Model file for the job. Use its own axes, mm. A direction names the side the tool comes from. Round coordinates to 2 decimals unless told otherwise and drop trailing zeros. Order: outer loops, then holes, each group sorted by start corner. A loop starts at its lowest first (then second) coordinate and runs counter-clockwise, first axis right, second up. Notation, with made-up numbers: (53, 68) - (106, 68) arc R17 ccw to (106, 84) - close; hole circle Ø6 at (-16.75, 88.25). An arc over 180 degrees is marked (long way). Answer as CSV lines item,"result". Start each with the question number.
1. Wall check: line 1 along Y through (x, z) = (31, 2.5); line 2 along Y through (x, z) = (-102.82, 1); line 3 along X through (y, z) = (21.5, 3.35). Give the ranges that are in metal, low to high. Write a range as [from, to].
2. Pull direction Y, two halves, no side cores. Call faces 1 (the face through (104.2, 13.6, 2)), 2 (the face through (33.03, 17, 2)), 3 (the face through (-9, 1, 0)): released by +Y, released by -Y, zero draft, split by the parting line, or undercut.
3. Band-saw the part on B-B on x = -37. List the corners of the cut face in (y, z), then the cut area to 3 significant figures.
4. Band-saw the part on A-A on x = -63.55. List the corners of the cut face in (y, z) (3 decimals), then the cut area to 3 significant figures.
5. Pin check, flat tip, straight feed: pin 1 Ø6 at (x, y) = (102.82, 15) entering from +Z. Stop position of the tip, or through.
6. Band-saw the part on C-C on z = 0.75. State how many separate pieces and enclosed holes the cut face has, then the cut area to 3 significant figures.
7. 3-axis set-ups, long thin cutter, end or side, ignore diameter. For faces 4 (the face through (-33.03, 18, 2)), 5 (the face through (-111, 23, 2)), 6 (the face through (-101, 28, 2)): which of +Z, -Z, +X, -X, +Y, -Y reach the whole face in a straight line?
8. Band-saw the part on D-D on x = 68. List the corners of the cut face in (y, z).
Autodesk Fusion 360 part; units mm, degrees
sketch "Sketch1" plane through (0, 0, 0) normal (0, 0, 1) x (1, 0, 0)
  line L0 (-111, 0.4) -> (111, 0.4)
  line L1 (111, 0.4) -> (111, 44.05)
  line L2 (111, 44.05) -> (-111, 44.05)
  line L3 (-111, 44.05) -> (-111, 0.4)
extrude "Extrude1" add sketch "Sketch1" along normal blind 4
sketch "Sketch2" plane through (0, 0, 0) normal (0, 0, 1) x (1, 0, 0)
  circle A0 centre (-63.55, 22.225) radius 19.5
  circle A1 centre (-79.55, 6.225) radius 1.8
  circle A2 centre (-79.55, 38.225) radius 1.8
  circle A3 centre (-47.55, 6.225) radius 1.8
  circle A4 centre (-47.55, 38.225) radius 1.8
  circle A5 centre (0, 22.225) radius 19.5
  circle A6 centre (-16, 6.225) radius 1.8
  circle A7 centre (-16, 38.225) radius 1.8
  circle A8 centre (16, 6.225) radius 1.8
  circle A9 centre (16, 38.225) radius 1.8
  circle A10 centre (63.55, 22.225) radius 19.5
  circle A11 centre (47.55, 6.225) radius 1.8
  circle A12 centre (47.55, 38.225) radius 1.8
  circle A13 centre (79.55, 6.225) radius 1.8
  circle A14 centre (79.55, 38.225) radius 1.8
  circle A15 centre (-102.82, 15) radius 1.7
  circle A16 centre (-102.82, 29.45) radius 1.7
  circle A17 centre (102.82, 15) radius 1.7
  circle A18 centre (102.82, 29.45) radius 1.7
extrude "Extrude2" cut sketch "Sketch2" along normal blind 4
sketch "Sketch3" plane through (0, 0, 0) normal (0, 0, 1) x (1, 0, 0)
  line L0 (-33.03, 15) -> (-30.53, 15)
  line L1 (-30.53, 15) -> (-30.53, 20)
  line L2 (-30.53, 20) -> (-33.03, 20)
  line L3 (-33.03, 20) -> (-33.03, 15)
  line L4 (-33.03, 24.5) -> (-30.53, 24.5)
  line L5 (-30.53, 24.5) -> (-30.53, 29.5)
  line L6 (-30.53, 29.5) -> (-33.03, 29.5)
  line L7 (-33.03, 29.5) -> (-33.03, 24.5)
  line L8 (30.53, 15) -> (33.03, 15)
  line L9 (33.03, 15) -> (33.03, 20)
  line L10 (33.03, 20) -> (30.53, 20)
  line L11 (30.53, 20) -> (30.53, 15)
  line L12 (30.53, 24.5) -> (33.03, 24.5)
  line L13 (33.03, 24.5) -> (33.03, 29.5)
  line L14 (33.03, 29.5) -> (30.53, 29.5)
  line L15 (30.53, 29.5) -> (30.53, 24.5)
  line L16 (88.19, 15) -> (90.69, 15)
  line L17 (90.69, 15) -> (90.69, 20)
  line L18 (90.69, 20) -> (88.19, 20)
  line L19 (88.19, 20) -> (88.19, 15)
  line L20 (88.19, 24.5) -> (90.69, 24.5)
  line L21 (90.69, 24.5) -> (90.69, 29.5)
  line L22 (90.69, 29.5) -> (88.19, 29.5)
  line L23 (88.19, 29.5) -> (88.19, 24.5)
extrude "Extrude3" cut sketch "Sketch3" along normal blind 4
ref_plane "WorkPlane1" through (0, 0, 4) normal (0, 0, 1) x (1, 0, 0)
sketch "Sketch4" plane through (0, 0, 4) normal (0, 0, 1) x (1, 0, 0)
  circle A0 centre (-102.82, 15) radius 3.25
  circle A1 centre (-102.82, 29.45) radius 3.25
  circle A2 centre (102.82, 15) radius 3.25
  circle A3 centre (102.82, 29.45) radius 3.25
extrude "Extrude4" cut sketch "Sketch4" against normal blind 2
sketch "Sketch5" plane through (0, 0, 0) normal (0, 0, 1) x (1, 0, 0)
  line L0 (-97.6, 2) -> (97.6, 2)
  line L1 (97.6, 2) -> (97.6, 4.4)
  line L2 (97.6, 4.4) -> (-97.6, 4.4)
  line L3 (-97.6, 4.4) -> (-97.6, 2)
  line L4 (-97.6, 40.05) -> (97.6, 40.05)
  line L5 (97.6, 40.05) -> (97.6, 42.45)
  line L6 (97.6, 42.45) -> (-97.6, 42.45)
  line L7 (-97.6, 42.45) -> (-97.6, 40.05)
extrude "Extrude5" cut sketch "Sketch5" along normal blind 2
Reply:
1,line 1,"y = [0.4, 15], [20, 24.5], [29.5, 44.05]"
1,line 2,"y = [0.4, 13.3], [16.7, 27.75], [31.15, 44.05]"
1,line 3,"x = [-111, -83.04], [-44.06, -19.49], [19.49, 44.06], [83.04, 111]"
2,face 1,"undercut"
2,face 2,"undercut"
2,face 3,"zero draft"
3,outline,"(0.4, 0) - (2, 0) - (2, 2) - (4.4, 2) - (4.4, 0) - (40.05, 0) - (40.05, 2) - (42.45, 2) - (42.45, 0) - (44.05, 0) - (44.05, 4) - (0.4, 4) - close"
3,area,"165 mm2"
4,outline,"(0.4, 0) - (2, 0) - (2, 2) - (2.725, 2) - (2.725, 4) - (0.4, 4) - close; (41.725, 2) - (42.45, 2) - (42.45, 0) - (44.05, 0) - (44.05, 4) - (41.725, 4) - close"
4,area,"15.7 mm2"
5,pin 1,"stops at z = 2"
6,separate pieces,"3"
6,enclosed holes,"23"
6,area,"5,040 mm2"
7,face 4,"+Z, -Z"
7,face 5,"+Z, -Z, -X, +Y, -Y"
7,face 6,"+Z"
8,outline,"(0.4, 0) - (2, 0) - (2, 2) - (3.24, 2) - (3.24, 4) - (0.4, 4) - close; (41.21, 2) - (42.45, 2) - (42.45, 0) - (44.05, 0) - (44.05, 4) - (41.21, 4) - close"
